Autodesk Inventor part; units mm, degrees
ref_plane "YZ Plane" through (0, 0, 0) normal (1, 0, 0) x (0, 1, 0)
ref_plane "XZ Plane" through (0, 0, 0) normal (0, 1, 0) x (-1, 0, 0)
ref_plane "XY Plane" through (0, 0, 0) normal (0, 0, 1) x (1, 0, 0)
sketch "Sketch1" plane through (0, 0, 0) normal (0, 1, 0) x (-1, 0, 0)
  line L0 (10, 3.5) -> (-4, 3.5)
  line L1 (-4, 3.5) -> (-4, -3.5)
  line L2 (-4, -3.5) -> (10, -3.5)
  line L3 (10, -3.5) -> (10, 3.5)
  line L4 (12.8, 0) -> (-6.8, 0)
  line L5 (0, -4.9) -> (0, 4.9)
  circle A0 centre (5, 0) radius 1
  dimension "d13" = 4
  dimension "d14" = 5
  dimension "d15" = 10
  dimension "d16" = 3.5
  dimension "d17" = 3.5
  dimension "d18" = 2
extrude "Extrusion4" add sketch "Sketch1" along normal blind 3 contours L3 L4 A0 L5 L0 | L5 L4 L1 L0 | L3 L2 L5 L4 A0 | L5 L2 L1 L4
sketch "Sketch3" plane through (0, 0, 0) normal (0, -1, 0) x (1, 0, 0)
  line L0 (4, -3.5) -> (-10, -3.5)
  line L1 (4, 3.5) -> (4, -3.5)
  line L2 (4, 3.5) -> (-1, 3.5)
  line L3 (-1, 3.5) -> (-1, -3.5)
  line L4 (-1, -3.5) -> (4, -3.5)
  line L5 (4, -3.5) -> (4, 3.5)
  point P0 (0, 0)
  dimension "d21" = 5
extrude "Extrusion5" add sketch "Sketch3" along normal blind 50
sketch "Sketch5" plane through (0, -50, 0) normal (0, -1, 0) x (1, 0, 0)
  line L0 (4, 3.5) -> (-1, 3.5)
  line L1 (-1, 3.5) -> (-1, -3.5)
  line L2 (-1, -3.5) -> (4, -3.5)
  line L3 (4, -3.5) -> (4, 3.5)
  line L4 (2.5, 3.5) -> (0.5, 3.5)
  line L5 (0.5, 3.5) -> (0.5, -3.5)
  line L6 (0.5, -3.5) -> (2.5, -3.5)
  line L7 (2.5, -3.5) -> (2.5, 3.5)
  point P0 (0, 0)
  dimension "d29" = 1.5
  dimension "d30" = 1.5
extrude "Extrusion7" add sketch "Sketch5" along normal blind 6 contours L7 L2 L5 L0
sketch "Sketch6" plane through (2.5, -50, 3.5) normal (1, 0, 0) x (0, 0, -1)
  circle A0 centre (3.5, -3) radius 1
  line L0 (7, 0) -> (0, 0)
  line L1 (0, 0) -> (0, -6)
  point P0 (3.5, 50)
  dimension "d34" = 2
  dimension "d35" = 3
  dimension "d36" = 3.5
extrude "Extrusion8" cut sketch "Sketch6" against normal through all
sketch "Sketch7" plane through (-1, 0, -3.5) normal (-1, 0, 0) x (0, 0, 1)
  line L0 (0, 0) -> (7, 0)
  line L1 (0, 0) -> (0, -50)
  line L2 (7, 0) -> (7, -50)
  line L3 (0, -4.05) -> (7, -4.05)
  line L4 (7, -4.05) -> (7, -8.05)
  line L5 (7, -8.05) -> (0, -8.05)
  line L6 (0, -8.05) -> (0, -4.05)
  point P0 (3.5, 0)
  dimension "d39" = 4.05
  dimension "d40" = 4
extrude "Extrusion9" add sketch "Sketch7" along normal blind 7.5 contours L3 L2 L5 L1
sketch "Sketch9" plane through (-1, -8.05, -3.5) normal (0, -1, 0) x (1, 0, 0)
  line L0 (0, 7) -> (-7.5, 7)
  line L1 (-7.5, 0) -> (-7.5, 7)
  line L2 (0, 0) -> (-7.5, 0)
  line L3 (-7.5, 0) -> (-2.5, 0)
  line L4 (-2.5, 0) -> (-2.5, 7)
  line L5 (-2.5, 7) -> (-7.5, 7)
  line L6 (-7.5, 7) -> (-7.5, 0)
  point P0 (1, 3.5)
  dimension "d43" = 5
extrude "Extrusion10" add sketch "Sketch9" along normal blind 50
sketch "Sketch10" plane through (-1, -50, -3.5) normal (-1, 0, 0) x (0, 0, 1)
  line L0 (7, 41.95) -> (0, 41.95)
  line L1 (0, 41.95) -> (0, 0)
  line L2 (7, 0) -> (0, 0)
  line L3 (7, 41.95) -> (7, 0)
  line L4 (0, 41.95) -> (10.2816, 41.95)
  line L5 (10.2816, 41.95) -> (10.2816, -15.7759)
  line L6 (10.2816, -15.7759) -> (0, -15.7759)
  line L7 (0, -15.7759) -> (0, 41.95)
  point P0 (3.5, 50)
extrude "Extrusion11" cut sketch "Sketch10" against normal blind 20
sketch "Sketch11" plane through (-1, -58.05, -3.5) normal (0, -1, 0) x (1, 0, 0)
  line L0 (-2.5, 7) -> (-7.5, 7)
  line L1 (-7.5, 7) -> (-7.5, 0)
  line L2 (-7.5, 0) -> (-2.5, 0)
  line L3 (-2.5, 0) -> (-2.5, 7)
  line L4 (-4, 0) -> (-6, 0)
  line L5 (-6, 0) -> (-6, 7)
  line L6 (-6, 7) -> (-4, 7)
  line L7 (-4, 7) -> (-4, 0)
  point P0 (1, 3.5)
  dimension "d48" = 1.5
  dimension "d49" = 1.5
extrude "Extrusion12" cut sketch "Sketch11" against normal blind 6 contours L3 L2 L7 L0 | L5 L2 L1 L0
sketch "Sketch12" plane through (-7, -58.05, -3.5) normal (-1, 0, 0) x (0, 0, 1)
  line L0 (7, 6) -> (7, 0)
  line L1 (7, 6) -> (0, 6)
  circle A0 centre (3.5, 3) radius 1
  point P0 (3.5, 58.05)
  dimension "d52" = 2
  dimension "d53" = 3.5
  dimension "d54" = 3
extrude "Extrusion13" cut sketch "Sketch12" against normal through all
thicken "Thicken1" operation add thickness 1 both sides no extend neighbours yes toward (1, 0, 0) faces at (-10, 1, -1.1667)
thicken "Thicken2" operation add thickness 0.5 both sides no extend neighbours yes toward (1, 0, 0) faces at (-9, 1, -1.1667)
properties part number "LD_holder_p3"
Here's how the part is built. I have some questions about the finished solid (model axes, mm). A direction names the side the tool comes from. Coordinates: 2 decimals unless noted, no trailing zeros. Loops run counter-clockwise (first coordinate to the right, second up) from the corner with the lowest first, then second, coordinate; pieces in that order, holes last. Notation, with made-up numbers: (0.5, 76) -> (25.5, 76) arc R27 ccw to (25.5, 92) -> close; hole circle Ø11 at (-4, 33). An arc over 180 degrees is marked (long way). Use one line per item in the form item = value. Start each with the question number.
(1) Will these pins go through, and if not, where does the flat tip stop? pin 1 (1 mm diameter, centred on x = 1.5, z = -0.5, fed in from -Y); pin 2 (0.8 mm diameter, centred on x = -4.5, z = -1, fed in from -Y); pin 3 (2.5 mm diameter, centred on y = -55.05, z = 0, fed in from -X); pin 4 (1.2 mm diameter, centred on x = -7.5, z = 1, fed in from -Y).
(2) We'd pull the mould along Y, two halves only. Please class faces 5 (the face through (-4, -20, -3.5)), 6 (the face through (-4, -52.05, 0)), 7 (the face through (-1, -2, 0)), 8 (the face through (-5, -4.05, 0)): pulls with the +Y half, pulls with the -Y half, needs draft (parallel to the pull), parting line crosses it, or undercut.
(3) If we section it at D-D (y = -39.5): Please give me the cut outline in (x, z).
(4) If we section it at A-A (y = -55.05): Please give me the cut outline in (x, z).
(5) Please list where these lines run through material, in increasing order: line 1 along Y through (x, z) = (-6.3, 0); line 2 along Y through (x, z) = (-3, 2.25); line 3 along Y through (x, z) = (-5.55, 0).
(6) If we section it at C-C (x = 3.25): Please give me the cut outline in (y, z), then the cut area to 4 significant figures.
(7) On a 3-axis mill with a long thin cutter (end or side, diameter ignored), from which of +Z, -Z, +X, -X, +Y, -Y can I reach the whole of each face in a straight line? I mean faces 1 (the face through (-4.2, 1.5, 0.6)), 2 (the face through (-4, 0, 1)), 3 (the face through (-3.5, -30, 0)), 4 (the face through (-8, -52.05, 0)). Say none if no direction works.
(8) If we section it at B-B (z = -2.75): Please give me the cut outline in (x, y), then the cut area to 3 significant figures.
Verdict:
q1.pin_1 = -8.05
q1.pin_2 = -52.05
q1.pin_3 = -7
q1.pin_4 = -58.05
q2.face_5 = needs draft
q2.face_6 = pulls with the -Y half
q2.face_7 = undercut
q2.face_8 = undercut
q3.outline = (-8.5, -3.5) -> (-3.5, -3.5) -> (-3.5, 3.5) -> (-8.5, 3.5) -> close
q4.outline = (-7, -3.5) -> (-5, -3.5) -> (-5, -1) -> (-7, -1) -> close; (-7, 1) -> (-5, 1) -> (-5, 3.5) -> (-7, 3.5) -> close
q5.line_1 = -58.05 to -56.05, -54.05 to -4.05, 0 to 3
q5.line_2 = -8.05 to -4.05, 0 to 3
q5.line_3 = -58.05 to -56.05, -54.05 to -4.05
q6.outline = (-8.05, -3.5) -> (3, -3.5) -> (3, 3.5) -> (-8.05, 3.5) -> close
q6.area = 77.35 mm²
q7.face_1 = +Y
q7.face_2 = +Z, -Z, -X
q7.face_3 = +Z, -Z, +X, -Y
q7.face_4 = +Z, -Z, -X, -Y
q8.outline = (-8.5, -52.05) -> (-7, -52.05) -> (-7, -58.05) -> (-5, -58.05) -> (-5, -52.05) -> (-3.5, -52.05) -> (-3.5, -8.05) -> (4, -8.05) -> (4, 3) -> (-8.5, 3) -> (-8.5, 0) -> (-1, 0) -> (-1, -4.05) -> (-8.5, -4.05) -> close
q8.area = 340 mm²
